Could you check a few things on this model? Use its own coordinates, in mm. Coordinates: 2 decimals unless noted, no trailing zeros. Order: outer loops, then holes, each group sorted by start corner. A loop starts at its lowest first (then second) coordinate and runs counter-clockwise, first axis right, second up. Notation, with made-up numbers: (87.5, -32) - (107.5, -32) arc R35 ccw to (107.5, 7) - close; hole circle Ø2 at (76, 29). An arc over 180 degrees is marked (long way). Answer as a JSON object with one key per item and string values. Group by question number.
(1) Imagine slicing it at C-C, the plane z = 0.3. Write out the boundary of the cut face in (x, y), and give its area (3 significant figures).
(2) Imagine slicing it at A-A, the plane y = 0. Write out the boundary of the cut face in (x, z), and give its area (3 significant figures).
(3) Imagine slicing it at D-D, the plane x = 0. Write out the boundary of the cut face in (y, z), and give its area (3 significant figures).
(4) Please list where these lines run through material, in increasing order: probe 1 along X at (y, z) = (0, 0.4); probe 2 along X at (y, z) = (2.5, 0.85); probe 3 along Y at (x, z) = (-3, 0.6).
(5) Imagine slicing it at B-B, the plane x = -1.5. Write out the boundary of the cut face in (y, z).
(6) Will these pins go through, and if not, where does the flat tip stop? P1, Ø5, axis at x = 0, y = 0, coming from the +Z side (3 decimals); P2, Ø1.5, axis at x = -4.5, y = -2.5, coming from the -Z side.
(7) We'd pull the mould along Y, two halves only. Please class faces 1 (the cylindrical face through (-5.717, 2.355, 0.493)), 2 (the flat face through (-3, 3, 1)), 3 (the cylindrical face through (-2.73, 4.19, 0.49)): pulls with the +Y half, pulls with the -Y half, needs draft (parallel to the pull), parting line crosses it, or undercut.
from build123d import *

# Parameters (mm, degrees)
CYLINDER004_R          = 1.5
CYLINDER004_DEPTH      = 1
CYLINDER002_R          = 1.5
CYLINDER002_DEPTH      = 1
CUT001_PLACEMENT_ANGLE = 318
MIRROR_PLACEMENT_ANGLE = 32
CYLINDER001_R          = 4
CYLINDER001_DEPTH      = 10
CYLINDER_R             = 5
CYLINDER_DEPTH         = 1


with BuildPart() as cylinder004:
    # Cylinder004 → Cylinder004 (new body)
    with BuildSketch(Plane(origin=(-5.5, 3.25, 0), x_dir=(1, 0, 0), z_dir=(0, 0, 1))):
        Circle(CYLINDER004_R)
    extrude(amount=CYLINDER004_DEPTH)


with BuildPart() as cut001:
    # Cylinder002 → Cylinder002 (new body)
    with BuildSketch(Plane(origin=(-5.5, 2, 0), x_dir=(1, 0, 0), z_dir=(0, 0, 1))):
        Circle(CYLINDER002_R)
    extrude(amount=CYLINDER002_DEPTH)

    # Cut001: cut Cylinder004
    add(cylinder004.part, mode=Mode.SUBTRACT)


with BuildPart() as cut001_1:
    # Cut001 placement: moved
    add(cut001.part.moved(Location((-2.5, -3, 0))).rotate(Axis((-2.5, -3, 0), (0, 0, 1)), CUT001_PLACEMENT_ANGLE))


with BuildPart() as cut001_mirrored:
    # Mirror: instance of Cut001
    add(cut001_1.part.mirror(Plane(origin=(-5.416318, 1.980722, 0), x_dir=(0.264078, -0.964501, 0), z_dir=(0.964501, 0.264078, 0))))


with BuildPart() as cut001_mirrored_1:
    # Mirror placement: moved
    add(cut001_mirrored.part.moved(Location((6, 7, 0))).rotate(Axis((6, 7, 0), (0, 0, 1)), MIRROR_PLACEMENT_ANGLE))


with BuildPart() as cylinder001:
    # Cylinder001 → Cylinder001 (new body)
    with BuildSketch(Plane.XY.offset(-5)):
        Circle(CYLINDER001_R)
    extrude(amount=CYLINDER001_DEPTH)


with BuildPart() as cut:
    # Cylinder → Cylinder (new body)
    with BuildSketch(Plane.XY):
        Circle(CYLINDER_R)
    extrude(amount=CYLINDER_DEPTH)

    # Cut: cut Cylinder001
    add(cylinder001.part, mode=Mode.SUBTRACT)


with BuildPart() as fusion:
    # Fusion base: copy of Cut001
    add(cut001_1.part)

    # Fusion: union Cut001 (mirrored), Cut
    add(cut001_mirrored_1.part)
    add(cut.part)


solid = fusion.part
Result set:
{
 "1": {"outline": "(-5.84, 3.54) arc R1.5 ccw to (-4.95, 0.7) arc R5 ccw (long way) to (1.3, 4.83) arc R1.5 ccw to (-0.83, 6.91) arc R1.5 cw to (0.34, 4.99) arc R5 ccw to (-4.73, 1.63) arc R1.5 cw to start; hole circle Ø8 at (0, 0)", "area": "34.4 mm^2"},
 "2": {"outline": "(-5, 0) - (-4, 0) - (-4, 1) - (-5, 1) - close; (4, 0) - (5, 0) - (5, 1) - (4, 1) - close", "area": "2.00 mm^2"},
 "3": {"outline": "(-5, 0) - (-4, 0) - (-4, 1) - (-5, 1) - close; (4, 0) - (5, 0) - (5, 1) - (4, 1) - close; (6.46, 0) - (7.24, 0) - (7.24, 1) - (6.46, 1) - close", "area": "2.79 mm^2"},
 "4": {"probe 1": "x = -5 to -4, 4 to 5", "probe 2": "x = -6.71 to -5.79, -4.33 to -3.12, 3.12 to 4.33", "probe 3": "y = -4 to -2.65, 2.65 to 4"},
 "5": {"outline": "(-4.77, 0) - (-3.71, 0) - (-3.71, 1) - (-4.77, 1) - close; (3.71, 0) - (4.77, 0) - (4.77, 1) - (3.71, 1) - close"},
 "6": {"P1": "passes through", "P2": "stops at z = 0"},
 "7": {"face 1": "undercut", "face 2": "needs draft", "face 3": "undercut"}
}
